Here's how the part is built. I have some questions about the finished solid (model axes, mm). A direction names the side the tool comes from. Coordinates: 2 decimals unless noted, no trailing zeros. Write each loop counter-clockwise with the first axis right and the second up, starting at its lowest first coordinate (ties: lowest second). Pieces come first, ordered by that corner, then holes. Notation, with made-up numbers: (-14.5, 88.25) -> (11.5, 88.25) arc R10 ccw to (11.5, 102.25) -> close; hole circle Ø8 at (84, -19.75). An arc over 180 degrees is marked (long way). Use a Markdown table: item, result. Add a question column.
Item 1: Imagine slicing it at D-D, the plane y = -7.5. Write out the boundary of the cut face in (x, z), and give its area (4 significant figures).
Item 2: On a 3-axis mill with a long thin cutter (end or side, diameter ignored), from which of +Z, -Z, +X, -X, +Y, -Y can I reach the whole of each face in a straight line? I mean faces 4 (the cylindrical face through (-15.475, -0.571, 4.93)), 5 (the cylindrical face through (10, 18, 5)), 6 (the flat face through (13, 18.5, 5)), 7 (the flat face through (-16, 14, 5)), 8 (the flat face through (16, 14, 5)). Say none if no direction works.
Item 3: Imagine slicing it at C-C, the plane x = 11. Write out the boundary of the cut face in (y, z), and give its area (3 significant figures).
Item 4: Imagine slicing it at B-B, the plane y = 11.5. Write out the boundary of the cut face in (x, z), and give its area (3 significant figures).
Item 5: If we mould it in two halves opening along X, with no side actions, what happens to faces 1 (the cylindrical face through (-16.26, 11.76, 5.07)), 2 (the flat face through (-12, 18.5, 5)), 3 (the flat face through (-9, 12, 5))? For each: pulls with the +X half, pulls with the -X half, needs draft (parallel to the pull), parting line crosses it, or undercut.
Item 6: Will these pins go through, and if not, where does the flat tip stop? pin 1 Ø12 at (x, y) = (8, -5) entering from +Z; pin 2 Ø4 at (y, z) = (4.5, 7) entering from +X; pin 3 Ø1.6 at (y, z) = (15, 3.5) entering from +X; pin 4 Ø3 at (x, z) = (-2, 5) entering from +Y.
Item 7: Imagine slicing it at A-A, the plane z = 5.25. Write out the boundary of the cut face in (x, y).
Item 8: If I drill on line 1 along Y through (x, z) = (-2, 9); line 2 along X through (y, z) = (-5, 4); line 3 along X through (y, z) = (-6, 2), over which ranges is the centre line in solid material (lowest first)? Write a range as from..to.
```python
from build123d import *

# Parameters (mm, degrees)
F1_DEPTH = 10
F2_R     = 2.5
F3_R     = 1


with BuildPart() as f1:
    # F0 (on Top) → F1 (new body)
    with BuildSketch(Plane.XY):
        with BuildLine():
            ThreePointArc((15.5, 0), (13.5961940777, -4.5961940777), (9, -6.5))
            Line((9, -6.5), (2.8321595662, -6.5))
            ThreePointArc((2.8321595662, -6.5), (1.5672713544, -8.4013556122), (0, -10.0623058987))
            ThreePointArc((0, -10.0623058987), (4.1829017881, -12.611326846), (9, -13.5))
            ThreePointArc((9, -13.5), (18.545941546, -9.545941546), (22.5, 0))
            ThreePointArc((22.5, 0), (20.763290356, 6.6238206497), (16, 11.5433963806))
            ThreePointArc((16, 11.5433963806), (12.634153881, 13.0016508786), (9, 13.5))
            Line((9, 13.5), (9, 6.5))
            ThreePointArc((9, 6.5), (13.5961940777, 4.5961940777), (15.5, 0))
        make_face()
        with BuildLine():
            ThreePointArc((0, -10.0623058987), (1.5672713544, -8.4013556122), (2.8321595662, -6.5))
            Line((2.8321595662, -6.5), (-2.8321595662, -6.5))
            ThreePointArc((-2.8321595662, -6.5), (-1.5672713544, -8.4013556122), (0, -10.0623058987))
        make_face()
        with BuildLine():
            Line((9, 18.5), (9, 13.5))
            ThreePointArc((9, 13.5), (12.634153881, 13.0016508786), (16, 11.5433963806))
            Line((16, 11.5433963806), (16, 18.5))
            Line((16, 18.5), (9, 18.5))
        make_face()
        with BuildLine():
            ThreePointArc((0, -10.0623058987), (-1.5672713544, -8.4013556122), (-2.8321595662, -6.5))
            Line((-2.8321595662, -6.5), (-9, -6.5))
            ThreePointArc((-9, -6.5), (-15.5, 0), (-9, 6.5))
            Line((-9, 6.5), (-9, 13.5))
            ThreePointArc((-9, 13.5), (-12.634153881, 13.0016508786), (-16, 11.5433963806))
            ThreePointArc((-16, 11.5433963806), (-22.0016508786, -3.634153881), (-9, -13.5))
            ThreePointArc((-9, -13.5), (-4.1829017881, -12.611326846), (0, -10.0623058987))
        make_face()
        with BuildLine():
            ThreePointArc((9, -13.5), (4.1829017881, -12.611326846), (0, -10.0623058987))
            ThreePointArc((0, -10.0623058987), (-4.1829017881, -12.611326846), (-9, -13.5))
            Line((-9, -13.5), (9, -13.5))
        make_face()
        with BuildLine():
            ThreePointArc((-16, 11.5433963806), (-12.634153881, 13.0016508786), (-9, 13.5))
            Line((-9, 13.5), (-9, 18.5))
            Line((-9, 18.5), (-16, 18.5))
            Line((-16, 18.5), (-16, 11.5433963806))
        make_face()
    extrude(amount=F1_DEPTH)

    # F2
    f2_edges = [f1.edges().sort_by_distance(p)[0] for p in [
        (16, 18.5, 5),
        (9, 18.5, 5),
        (-9, 18.5, 5),
        (-16, 18.5, 5),
        (16, 11.543396, 5),
        (-16, 11.543396, 5),
    ]]
    fillet(f2_edges, radius=F2_R)

    # F3
    f3_edges = [f1.edges().sort_by_distance(p)[0] for p in [
        (-9, -6.5, 5),
        (9, -6.5, 5),
        (-9, 6.5, 5),
        (9, 6.5, 5),
    ]]
    fillet(f3_edges, radius=F3_R)


solid = f1.part
```
Ans:
| question | item | result |
|---|---|---|
| 1 | outline | (-20.22, 0) -> (20.22, 0) -> (20.22, 10) -> (-20.22, 10) -> close |
| 1 | area | 404.5 mm^2 |
| 2 | face 4 | +Z, -Z |
| 2 | face 5 | +Z, -Z, +Y |
| 2 | face 6 | +Z, -Z, +X, -X, +Y |
| 2 | face 7 | +Z, -Z, -X, +Y |
| 2 | face 8 | +Z, -Z, +X, +Y |
| 3 | outline | (-13.35, 0) -> (-6.18, 0) -> (-6.18, 10) -> (-13.35, 10) -> close; (6.18, 0) -> (18.45, 0) -> (18.45, 10) -> (6.18, 10) -> close |
| 3 | area | 194 mm^2 |
| 4 | outline | (-16.41, 0) -> (-9, 0) -> (-9, 10) -> (-16.41, 10) -> close; (9, 0) -> (16.41, 0) -> (16.41, 10) -> (9, 10) -> close |
| 4 | area | 148 mm^2 |
| 5 | face 1 | pulls with the -X half |
| 5 | face 2 | needs draft |
| 5 | face 3 | undercut |
| 6 | pin 1 | stops at z = 10 |
| 6 | pin 2 | stops at x = 22.27 |
| 6 | pin 3 | stops at x = 16 |
| 6 | pin 4 | stops at y = -6.5 |
| 7 | outline | (-17.02, 10.86) arc R13.5 ccw to (-9, -13.5) -> (9, -13.5) arc R13.5 ccw to (17.02, 10.86) arc R2.5 cw to (16, 12.87) -> (16, 16) arc R2.5 ccw to (13.5, 18.5) -> (11.5, 18.5) arc R2.5 ccw to (9, 16) -> (9, 7.43) arc R1 ccw to (9.87, 6.44) arc R6.5 cw to (9, -6.5) -> (-9, -6.5) arc R6.5 cw to (-9.87, 6.44) arc R1 ccw to (-9, 7.43) -> (-9, 16) arc R2.5 ccw to (-11.5, 18.5) -> (-13.5, 18.5) arc R2.5 ccw to (-16, 16) -> (-16, 12.87) arc R2.5 cw to start |
| 8 | line 1 | y = -13.5..-6.5 |
| 8 | line 2 | x = -21.54..-13.15, 13.15..21.54 |
| 8 | line 3 | x = -21.09..-11.5, 11.5..21.09 |
